Can you work these out from the model? Positions are in its coordinate system, mm. A direction names the side the tool comes from. Coordinates: 2 decimals unless noted, no trailing zeros. Order: outer loops, then holes, each group sorted by start corner. A loop starts at its lowest first (then second) coordinate and runs counter-clockwise, first axis right, second up. Notation, with made-up numbers: M 25.5,7.5 L 68.5,7.5 A22 ccw 68.5,13.5 Z; hole C 45.25,42.5 d10. An arc over 180 degrees is marked long. Answer as CSV lines item,"result". Start each with the question number.
1. If we section it at B-B (y = -57.25): List the corners of the cut face in (x, z) for me.
2. I need wall thicknesses on line 1 along Z through (x, y) = (0, -53.5); line 2 along X through (y, z) = (-53.35, 349.5); line 3 along X through (y, z) = (-56.25, 310.5). Which ranges of each line are inside material? Lowest first, please. Write a range as from..to.
3. Will these pins go through, and if not, where does the flat tip stop? pin 1 (4 mm diameter, centred on x = 2, z = 348, fed in from -Y); pin 2 (3.5 mm diameter, centred on x = 0, z = 349.5, fed in from -Y); pin 3 (1 mm diameter, centred on x = 4.5, y = -54.5, fed in from +Z); pin 4 (6 mm diameter, centred on x = -1, z = 349, fed in from -Y).
4. If we section it at A-A (z = 330): List the corners of the cut face in (x, y) for me (3 decimals).
5. On a 3-axis mill with a long thin cutter (end or side, diameter ignored), from which of +Z, -Z, +X, -X, +Y, -Y can I reach the whole of each face in a straight line? I mean faces 1 (the face through (0.099, -54.018, 308.252)), 2 (the face through (1.262, -56.518, 314.506)). Say none if no direction works.
6. If we mould it in two halves opening along X, with no side actions, what happens to faces 3 (the face through (-4, -57.75, 330)), 4 (the face through (-6.5, -55, 330)), 5 (the face through (-2, -55.25, 312))? For each: released by +X, released by -X, zero draft, split by the parting line, or undercut.
7. If we section it at D-D (z = 348): List the corners of the cut face in (x, y) for me.
8. If we section it at C-C (x = 0.75): List the corners of the cut face in (y, z) for me, plus the area to 3 significant figures.
```python
from build123d import *

# Parameters (mm, degrees)
BARRA_START         = -57.75
SK_BARRA_W          = 13
SK_BARRA_H          = 39
BARRA_DEPTH         = 5
EXTREMOS_START      = -57.75
SK_EXTREMOS_R       = 6.5
EXTREMOS_DEPTH      = 5
PERNO_696_START     = -64.75
SK_PERNO_696_R      = 2.975
PERNO_696_DEPTH     = 7
PASANTES_M4_START   = -57.75
SK_PASANTES_M4_R    = 2.25
PASANTES_M4_DEPTH   = 5
AVELLANADO_M4_START = -57.75
SK_AVELLANADO_M4_R  = 4.2
AVELLANADO_M4_DEPTH = 2.5


with BuildPart() as part:
    # Sk_Barra → Barra (new body)
    with BuildSketch(Plane(origin=(0, 0, 0), x_dir=(1, 0, 0), z_dir=(0, 1, 0)).offset(BARRA_START)):
        with Locations((0, -330)):
            Rectangle(SK_BARRA_W, SK_BARRA_H)
    extrude(amount=BARRA_DEPTH)

    # Sk_Extremos → Extremos (add)
    with BuildSketch(Plane(origin=(0, 0, 0), x_dir=(1, 0, 0), z_dir=(0, 1, 0)).offset(EXTREMOS_START)):
        with Locations((0, -310.5)):
            Circle(SK_EXTREMOS_R)
        with Locations((0, -349.5)):
            Circle(SK_EXTREMOS_R)
    extrude(amount=EXTREMOS_DEPTH)

    # Sk_Perno_696 → Perno_696 (add)
    with BuildSketch(Plane(origin=(0, 0, 0), x_dir=(1, 0, 0), z_dir=(0, 1, 0)).offset(PERNO_696_START)):
        with Locations(Location((0, -330, 0), (0, 0, 270))):
            Circle(SK_PERNO_696_R)
    extrude(amount=PERNO_696_DEPTH)

    # Sk_Pasantes_M4 → Pasantes_M4 (cut)
    with BuildSketch(Plane(origin=(0, 0, 0), x_dir=(1, 0, 0), z_dir=(0, 1, 0)).offset(PASANTES_M4_START)):
        with Locations(Location((0, -310.5, 0), (0, 0, 270))):
            Circle(SK_PASANTES_M4_R)
        with Locations(Location((0, -349.5, 0), (0, 0, 270))):
            Circle(SK_PASANTES_M4_R)
    extrude(amount=PASANTES_M4_DEPTH, mode=Mode.SUBTRACT)

    # Sk_Avellanado_M4 → Avellanado_M4 (cut)
    with BuildSketch(Plane(origin=(0, 0, 0), x_dir=(1, 0, 0), z_dir=(0, 1, 0)).offset(AVELLANADO_M4_START)):
        with Locations(Location((0, -310.5, 0), (0, 0, 270))):
            Circle(SK_AVELLANADO_M4_R)
        with Locations(Location((0, -349.5, 0), (0, 0, 270))):
            Circle(SK_AVELLANADO_M4_R)
    extrude(amount=AVELLANADO_M4_DEPTH, mode=Mode.SUBTRACT)


solid = part.part
```
Solved:
1,outline,"M -6.5,310.5 A6.5 ccw 6.5,310.5 L 6.5,349.5 A6.5 ccw -6.5,349.5 Z; hole C 0,310.5 d8.4; hole C 0,349.5 d8.4"
2,line 1,"304..308.25, 312.75..347.25, 351.75..356"
2,line 2,"-6.5..-2.25, 2.25..6.5"
2,line 3,"-6.5..-4.2, 4.2..6.5"
3,pin 1,"y = -57.75"
3,pin 2,"through"
3,pin 3,"z = 354.62"
3,pin 4,"y = -55.25"
4,outline,"M -6.5,-57.75 L -2.975,-57.75 L -2.975,-64.75 L 2.975,-64.75 L 2.975,-57.75 L 6.5,-57.75 L 6.5,-52.75 L -6.5,-52.75 Z"
5,face 1,"+Y, -Y"
5,face 2,"-Y"
6,face 3,"zero draft"
6,face 4,"released by -X"
6,face 5,"undercut"
7,outline,"M -6.5,-57.75 L -3.92,-57.75 L -3.92,-55.25 L -1.68,-55.25 L -1.68,-52.75 L -6.5,-52.75 Z; M 1.68,-55.25 L 3.92,-55.25 L 3.92,-57.75 L 6.5,-57.75 L 6.5,-52.75 L 1.68,-52.75 Z"
8,outline,"M -64.75,327.12 L -57.75,327.12 L -57.75,314.63 L -55.25,314.63 L -55.25,312.62 L -52.75,312.62 L -52.75,347.38 L -55.25,347.38 L -55.25,345.37 L -57.75,345.37 L -57.75,332.88 L -64.75,332.88 Z; M -57.75,304.04 L -52.75,304.04 L -52.75,308.38 L -55.25,308.38 L -55.25,306.37 L -57.75,306.37 Z; M -57.75,353.63 L -55.25,353.63 L -55.25,351.62 L -52.75,351.62 L -52.75,355.96 L -57.75,355.96 Z"
8,area,"237 mm²"
